Design review of the part shown in the three views and the two pictorial views. Dimensions are in mm from the part's minimum x, y and z. A direction names the side the tool comes from. Coordinates: 2 decimals unless noted, no trailing zeros. Loops run counter-clockwise (first coordinate to the right, second up) from the corner with the lowest first, then second, coordinate; pieces in that order, holes last. Notation, with made-up numbers: (-27, 30) -> (23, 30) arc R13 ccw to (23, 43) -> close; hole circle Ø3 at (21.25, -16.75). An arc over 180 degrees is marked (long way). Use CSV: the item, a comma, the result in double quotes.
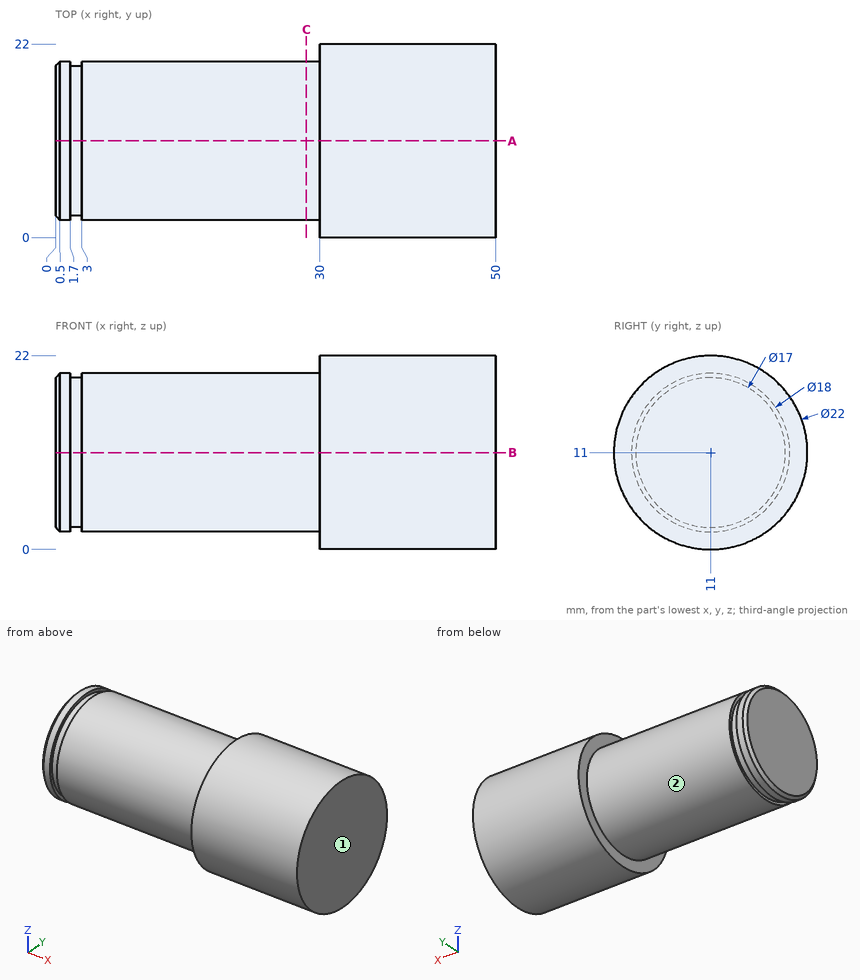
Item 1: Clearance check with flat-ended pins moving along their axes: pin 1 (12 mm diameter, centred on x = 7, z = 16.5, fed in from +Y); pin 2 (6 mm diameter, centred on x = 36.5, y = 5, fed in from +Z); pin 3 (12 mm diameter, centred on x = 19, z = 12, fed in from -Y). State where each tip first meets the part, or that it passes through.
Checked values:
pin 1,"y = 20"
pin 2,"z = 21.58"
pin 3,"y = 2"
Item 2: Machinability: for the marked faces 1 and 2, which of the approach directions +Z, -Z, +X, -X, +Y, -Y give a long, thin tool a straight path to every point of the face, cutting with its end or side? Answer none if there is none.
Checked values:
face 1,"+Z, -Z, +X, +Y, -Y"
face 2,"-X"
Item 3: To check wall thickness, follow line 1 along X through (y, z) = (18, 3.5); line 2 along X through (y, z) = (4, 16.25); line 3 along Z through (x, y) = (7, 7.75). State the ranges of each line that lie inside material, in increasing order.
Checked values:
line 1,"30 to 50"
line 2,"0.25 to 1.7, 3 to 50"
line 3,"2.61 to 19.39"
Item 4: Add section C-C (x = 28.5). Give the boundary of the cut face in (y, z).
Checked values:
outline,"circle Ø18 at (11, 11)"
Item 5: Add section A-A (y = 11). Give the boundary of the cut face in (x, z), then the cut area to 3 significant figures.
Checked values:
outline,"(0, 2.5) -> (0.5, 2) -> (1.7, 2) -> (1.7, 2.5) -> (3, 2.5) -> (3, 2) -> (30, 2) -> (30, 0) -> (50, 0) -> (50, 22) -> (30, 22) -> (30, 20) -> (3, 20) -> (3, 19.5) -> (1.7, 19.5) -> (1.7, 20) -> (0.5, 20) -> (0, 19.5) -> close"
area,"978 mm^2"
